Part model, mm, in its own coordinate system. Face numbers are marked on the shaded views. A direction names the side the tool comes from. Coordinates: 2 decimals unless noted, no trailing zeros. Loops run counter-clockwise (first coordinate to the right, second up) from the corner with the lowest first, then second, coordinate; pieces in that order, holes last. Notation, with made-up numbers: M 50.5,-31 L 109.5,-31 A26 cw 109.5,1 Z; hole C 24.25,-29.75 d3. An arc over 180 degrees is marked long. Use a Markdown table: item, result. Add a question column.
1) Wall check: probe 1 along X at (y, z) = (-1.25, 0); probe 2 along Y at (x, z) = (21.5, -3); probe 3 along X at (y, z) = (-2.5, 3.5). Give the ranges that are in metal, low to high. Write a range as from..to.
2) Band-saw the part on A-A (y = 1.25). List the corners of the cut face in (x, z).
3) Band-saw the part on D-D (y = -4.25). List the corners of the cut face in (x, z).
4) Band-saw the part on B-B (z = 0). List the corners of the cut face in (x, y).
5) Pull direction Z, two halves, no side cores. Call the marked faces 4, 5 and 6: released by +Z, released by -Z, zero draft, split by the parting line, or undercut.
6) Tool access for the marked faces 1, 2 and 3: list every direction of +Z, -Z, +X, -X, +Y, -Y with a clear straight run to the whole face (end or side of a thin tool).
7) Band-saw the part on C-C (x = 21). List the corners of the cut face in (y, z).
8) Pin check, flat tips, straight feed: pin 1 Ø6 at (y, z) = (3.5, 5.5) entering from -X; pin 2 Ø5 at (y, z) = (2.5, 4.5) entering from +X; pin 3 Ø6 at (x, y) = (10.5, -1.5) entering from -Z. Stop position of each tip, or through.
from build123d import *

# Parameters (mm, degrees)
SKETCH3_R           = 7
SKETCH3_R_2         = 2
BOSS_EXTRUDE1_DEPTH = 5


with BuildPart() as part:
    # Sketch2 → Revolve1 (revolve)
    with BuildSketch(Plane.XY, mode=Mode.PRIVATE) as revolve1_sk:
        Polygon((5.5, 0), (10, 0), (10, -9), (5.5, -6.5), align=None)
    revolve(revolve1_sk.sketch.rotate(Axis((0, 0, 0), (0, 1, 0)), 90), axis=Axis((0, 0, 0), (0, 1, 0)))

    # Sketch3 → Boss-Extrude1 (add)
    with BuildSketch(Plane(origin=(0, 0, 0), x_dir=(1, 0, 0), z_dir=(0, 1, 0))):
        with BuildLine():
            Line((-0.780909149, 12.835767591), (-25.956866437, 1.756247881))
            ThreePointArc((-25.956866437, 1.756247881), (-27, 0), (-25.956866437, -1.756247881))
            Line((-25.956866437, -1.756247881), (-0.780909149, -12.835767591))
            ThreePointArc((-0.780909149, -12.835767591), (-0.398996047, -12.958497669), (0, -13))
            ThreePointArc((0, -13), (0.398996047, -12.958497669), (0.780909149, -12.835767591))
            Line((0.780909149, -12.835767591), (25.956866437, -1.756247881))
            ThreePointArc((25.956866437, -1.756247881), (27, 0), (25.956866437, 1.756247881))
            Line((25.956866437, 1.756247881), (0.780909149, 12.835767591))
            ThreePointArc((0.780909149, 12.835767591), (0.398996047, 12.958497669), (0, 13))
            ThreePointArc((0, 13), (-0.398996047, 12.958497669), (-0.780909149, 12.835767591))
        make_face()
        with Locations(Location((0, 0, 0), (0, 0, 270))):
            Circle(SKETCH3_R, mode=Mode.SUBTRACT)
        with Locations(Location((21.5, 0, 0), (0, 0, 270))):
            Circle(SKETCH3_R_2, mode=Mode.SUBTRACT)
        with Locations(Location((-21.5, 0, 0), (0, 0, 270))):
            Circle(SKETCH3_R_2, mode=Mode.SUBTRACT)
    extrude(amount=BOSS_EXTRUDE1_DEPTH)


solid = part.part
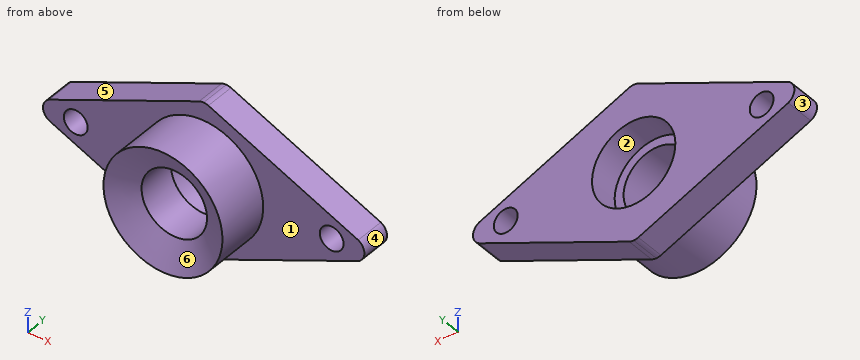
Entries:
| question | item | result |
|---|---|---|
| 1 | probe 1 | -10..-5.5, 5.5..10 |
| 1 | probe 2 | 0..5 |
| 1 | probe 3 | -9.37..-4.24, 4.24..9.37 |
| 2 | outline | M -25.96,-1.76 L -0.78,-12.84 A1.94 ccw 0.78,-12.84 L 25.96,-1.76 A2 ccw 25.96,1.76 L 0.78,12.84 A1.94 ccw -0.78,12.84 L -25.96,1.76 A2 ccw Z; hole C -21.5,0 d4; hole C 0,0 d14; hole C 21.5,0 d4 |
| 3 | outline | C 0,0 d20; hole C 0,0 d11 |
| 4 | outline | M -27,0 L -23.5,0 L -23.5,5 L -27,5 Z; M -19.5,0 L -10,0 L -10,-9 L -5.5,-6.5 L -5.5,0 L -7,0 L -7,5 L -19.5,5 Z; M 5.5,-6.5 L 10,-9 L 10,0 L 19.5,0 L 19.5,5 L 7,5 L 7,0 L 5.5,0 Z; M 23.5,0 L 27,0 L 27,5 L 23.5,5 Z |
| 5 | face 4 | split by the parting line |
| 5 | face 5 | released by +Z |
| 5 | face 6 | undercut |
| 6 | face 1 | -Y |
| 6 | face 2 | +Y |
| 6 | face 3 | -X, +Y, -Y |
| 7 | outline | M 0,-3.94 L 5,-3.94 L 5,-1.94 L 0,-1.94 Z; M 0,1.94 L 5,1.94 L 5,3.94 L 0,3.94 Z |
| 8 | pin 1 | x = -24.27 |
| 8 | pin 2 | x = 25.4 |
| 8 | pin 3 | z = -9.7 |
